Autodesk Inventor part; units mm, degrees
ref_plane "YZ Plane" through (0, 0, 0) normal (1, 0, 0) x (0, 1, 0)
ref_plane "XZ Plane" through (0, 0, 0) normal (0, 1, 0) x (-1, 0, 0)
ref_plane "XY Plane" through (0, 0, 0) normal (0, 0, 1) x (1, 0, 0)
sketch "Sketch1" plane through (0, 0, 0) normal (1, 0, 0) x (0, 1, 0)
  line L0 (0, 0) -> (9, 0)
  line L1 (9, 0) -> (9, -10)
  line L2 (9, -10) -> (10, -10)
  line L3 (10, -10) -> (10, -30)
  line L4 (10, -30) -> (6, -30)
  line L5 (6, -30) -> (6, -45)
  line L6 (6, -45) -> (10, -45)
  line L7 (10, -45) -> (10, -50)
  line L8 (0, 0) -> (0, -125)
  line L9 (10, -50) -> (4.5, -50)
  line L10 (4.5, -50) -> (4.5, -54)
  line L11 (4.5, -54) -> (7, -54)
  line L12 (7, -54) -> (7, -125)
  line L13 (7, -125) -> (0, -125)
  dimension "d1" = 18
  dimension "d2" = 20
  dimension "d3" = 12
  dimension "d4" = 20
  dimension "d5" = 9
  dimension "d6" = 14
  dimension "d7" = 20
  dimension "d8" = 15
  dimension "d9" = 4
  dimension "d10" = 5
  dimension "d11" = 71
  dimension "d12" = 125
revolve "Revolution1" add sketch "Sketch1" angle 360 about axis through (0, 0, 0) along (0, 0, -1)
thread "Thread1"
hole "Hole1" at (0, 0, 0) direction (0, 0, -1) diameter 4 depth 3 tip angle 118
sketch "Sketch2" plane through (0, 0, -125) normal (0, 0, -1) x (-1, 0, 0)
  point P0 (0, 0)
  point P1 (0, 0)
hole "Hole2" at (0, 0, -125) direction (0, 0, 1) diameter 4 depth 3 tip angle 118
chamfer "Chamfer1" distance 1 angle 45 9 edges at (0, -9, 0) (0, 2, 0) (0, -10, -10) (0, -10, -45) (0, -10, -50) (0, -7, -54) (0, -7, -125) (0, -2, -125) (0, -10, -30)
fillet "Fillet1" radius 1 1 edges at (0, -6, -30)
properties part number "b7"
For this review, take the finished solid that the model builds, in its own axes (mm). A direction names the side the tool comes from. Round coordinates to 2 decimals unless told otherwise and drop trailing zeros. Loops run counter-clockwise (first coordinate to the right, second up) from the corner with the lowest first, then second, coordinate; pieces in that order, holes last. Notation, with made-up numbers: (43.5, 76) - (71.5, 76) arc R28 ccw to (71.5, 106) - close; hole circle Ø7 at (52, -40). An arc over 180 degrees is marked (long way). Use one line per item in the form item = value.
1) Tool access review of faces 4 (the face through (4.5, -1.4, -54)), 5 (the face through (-2.681, 6.466, -89.983)), 6 (the face through (8.923, -1.172, -5.563)): name each direction out of +Z, -Z, +X, -X, +Y, -Y from which nothing blocks a thin tool from reaching the whole face with its end or side.
Solutions:
face_4 = none
face_5 = -Z
face_6 = +Z
2) Wall thickness on probe 1 along X at (y, z) = (0, -123.4); probe 2 along Z at (x, y) = (-5.5, -1); probe 3 along Z at (x, y) = (3.75, -5): over which ranges is each line inside the solid? List them lowest first.
Solutions:
probe_1 = -7 to -2, 2 to 7
probe_2 = -125 to -54, -50 to 0
probe_3 = -124.75 to -54.25, -50 to -45, -30.34 to 0
3) Clearance check with flat-ended pins moving along their axes: P1, Ø10, axis at x = 1, z = -79.5, coming from the -Y side; P2, Ø1.5, axis at y = 7, z = -33.5, coming from the -X side; P3, Ø1, axis at y = 2.5, z = -61.5, coming from the -X side; P4, Ø4, axis at x = -5, z = -72.5, coming from the +Y side. State where each tip first meets the part, or that it passes through.
Solutions:
P1 = -7
P2 = through
P3 = -6.71
P4 = 6.32
4) We need section A-A on z = -25. Write out the cut boundary in (x, y).
Solutions:
outline = circle Ø20 at (0, 0)
5) We need section B-B on z = -75.5. Write out the cut boundary in (x, y).
Solutions:
outline = circle Ø14 at (0, 0)
6) Mouldability with a two-part tool opening along Z and no side actions: class faces 1 (the face through (0.1, 3.4, 0)), 2 (the face through (2, 0, -2)), 3 (the face through (-6, 2, -45)) as pulls with the +Z half, pulls with the -Z half, needs draft (parallel to the pull), parting line crosses it, or undercut.
Solutions:
face_1 = pulls with the +Z half
face_2 = needs draft
face_3 = undercut
